Source: CAD feature listing. Evaluate the final solid. Frame: model axes, mm. Face numbers are marked on the shaded views. A direction names the side the tool comes from. Give positions to 0.01 mm unless a question says otherwise; leave off trailing zeros. Loops run counter-clockwise (first coordinate to the right, second up) from the corner with the lowest first, then second, coordinate; pieces in that order, holes last. Notation, with made-up numbers: (-25.5, 73.25) -> (-10.5, 73.25) arc R24 cw to (-10.5, 90.25) -> close; hole circle Ø4 at (-19, 31). An arc over 180 degrees is marked (long way). Return JSON: item names as keys, results as strings. Group by question number.
(1) Cut plane A-A on z = 0. Return loops of the section in (x, y), then the cut area to 3 significant figures.
(2) Pin query (flat end, axial travel): pin 1 (3 mm diameter, centred on y = 0, z = 0, fed in from +X). Return the tip coordinate at first contact, or that it passes through.
(3) Cut plane C-C on y = 4.25. Return loops of the section in (x, z), then the cut area to 3 significant figures.
(4) Ray query, line 1 (Y direction, x = 2.4, z = 0); line 2 (Z direction, x = 0.9, y = 0); line 3 (Z direction, x = 2.8, y = -3.75). Return the intervals inside material, ascending. Write a range as from..to.
(5) Draft query along Y for the marked faces 6, 7 and 8. Return one class per face: released by +Y, released by -Y, zero draft, split by the parting line, or undercut.
(6) Cut plane B-B on y = 0. Return loops of the section in (x, z), then the cut area to 3 significant figures.
(7) Access query for the marked faces 1, 2, 3, 4 and 5. Directions: +Z, -Z, +X, -X, +Y, -Y. A direction counts if a zero-diameter tool reaches every point of the face in a straight line with its end or side. Return the directions, or none.
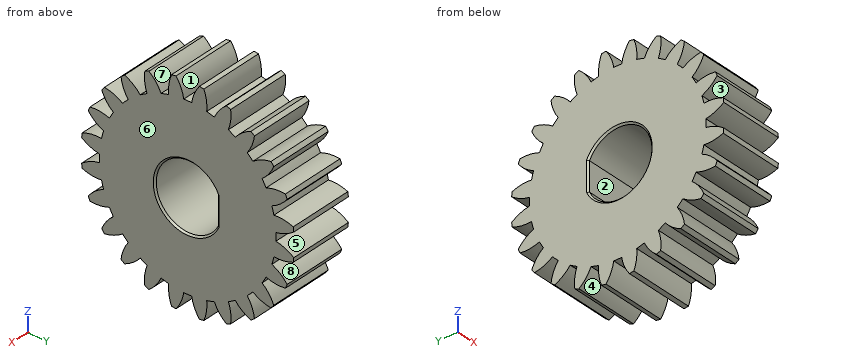
```python
from build123d import *

# Parameters (mm, degrees)
EXTRUDE_1_DEPTH = 4
CHAMFER_1_SIZE  = 0.1


with BuildPart() as part:
    # 草图1 → 凸台-拉伸1 (new body)
    with BuildSketch(Plane(origin=(0, 0, 0), x_dir=(0, -1, 0), z_dir=(-1, 0, 0))):
        with BuildLine():
            ThreePointArc((-0.711337602, 6.460959589), (-0.848420249, 6.444391599), (-0.98512003, 6.424915449))
            ThreePointArc((-0.98512003, 6.424915449), (-1.144628565, 5.84730165), (-1.156074481, 5.248177569))
            ThreePointArc((-1.156074481, 5.248177569), (-1.390893548, 5.19088539), (-1.622898915, 5.123092339))
            ThreePointArc((-1.622898915, 5.123092339), (-1.93237341, 5.636226055), (-2.359318752, 6.056700011))
            ThreePointArc((-2.359318752, 6.056700011), (-2.48744231, 6.005216961), (-2.614443361, 5.951023938))
            ThreePointArc((-2.614443361, 5.951023938), (-2.619019322, 5.351808006), (-2.475010506, 4.770136161))
            ThreePointArc((-2.475010506, 4.770136161), (-2.687, 4.65402052), (-2.893553842, 4.528490053))
            ThreePointArc((-2.893553842, 4.528490053), (-3.325292028, 4.944041268), (-3.846516229, 5.239686336))
            ThreePointArc((-3.846516229, 5.239686336), (-3.956949289, 5.156796712), (-4.065596697, 5.071579981))
            ThreePointArc((-4.065596697, 5.071579981), (-3.91492824, 4.49159749), (-3.625278654, 3.967017857))
            ThreePointArc((-3.625278654, 3.967017857), (-3.799991842, 3.799991842), (-3.967017857, 3.625278654))
            ThreePointArc((-3.967017857, 3.625278654), (-4.49159749, 3.91492824), (-5.071579981, 4.065596697))
            ThreePointArc((-5.071579981, 4.065596697), (-5.156796712, 3.956949289), (-5.239686336, 3.846516229))
            ThreePointArc((-5.239686336, 3.846516229), (-4.944041268, 3.325292028), (-4.528490053, 2.893553842))
            ThreePointArc((-4.528490053, 2.893553842), (-4.65402052, 2.687), (-4.770136161, 2.475010506))
            ThreePointArc((-4.770136161, 2.475010506), (-5.351808006, 2.619019322), (-5.951023938, 2.614443361))
            ThreePointArc((-5.951023938, 2.614443361), (-6.005216961, 2.48744231), (-6.056700011, 2.359318752))
            ThreePointArc((-6.056700011, 2.359318752), (-5.636226055, 1.93237341), (-5.123092339, 1.622898915))
            ThreePointArc((-5.123092339, 1.622898915), (-5.19088539, 1.390893548), (-5.248177569, 1.156074481))
            ThreePointArc((-5.248177569, 1.156074481), (-5.84730165, 1.144628565), (-6.424915449, 0.98512003))
            ThreePointArc((-6.424915449, 0.98512003), (-6.444391599, 0.848420249), (-6.460959589, 0.711337602))
            ThreePointArc((-6.460959589, 0.711337602), (-5.94431135, 0.407766737), (-5.368564348, 0.241646108))
            ThreePointArc((-5.368564348, 0.241646108), (-5.374, 0), (-5.368564348, -0.241646108))
            ThreePointArc((-5.368564348, -0.241646108), (-5.94431135, -0.407766737), (-6.460959589, -0.711337602))
            ThreePointArc((-6.460959589, -0.711337602), (-6.444391599, -0.848420249), (-6.424915449, -0.98512003))
            ThreePointArc((-6.424915449, -0.98512003), (-5.84730165, -1.144628565), (-5.248177569, -1.156074481))
            ThreePointArc((-5.248177569, -1.156074481), (-5.19088539, -1.390893548), (-5.123092339, -1.622898915))
            ThreePointArc((-5.123092339, -1.622898915), (-5.636226055, -1.93237341), (-6.056700011, -2.359318752))
            ThreePointArc((-6.056700011, -2.359318752), (-6.005216961, -2.48744231), (-5.951023938, -2.614443361))
            ThreePointArc((-5.951023938, -2.614443361), (-5.351808006, -2.619019322), (-4.770136161, -2.475010506))
            ThreePointArc((-4.770136161, -2.475010506), (-4.65402052, -2.687), (-4.528490053, -2.893553842))
            ThreePointArc((-4.528490053, -2.893553842), (-4.944041268, -3.325292028), (-5.239686336, -3.846516229))
            ThreePointArc((-5.239686336, -3.846516229), (-5.156796712, -3.956949289), (-5.071579981, -4.065596697))
            ThreePointArc((-5.071579981, -4.065596697), (-4.49159749, -3.91492824), (-3.967017857, -3.625278654))
            ThreePointArc((-3.967017857, -3.625278654), (-3.799991842, -3.799991842), (-3.625278654, -3.967017857))
            ThreePointArc((-3.625278654, -3.967017857), (-3.91492824, -4.49159749), (-4.065596697, -5.071579981))
            ThreePointArc((-4.065596697, -5.071579981), (-3.956949289, -5.156796712), (-3.846516229, -5.239686336))
            ThreePointArc((-3.846516229, -5.239686336), (-3.325292028, -4.944041268), (-2.893553842, -4.528490053))
            ThreePointArc((-2.893553842, -4.528490053), (-2.687, -4.65402052), (-2.475010506, -4.770136161))
            ThreePointArc((-2.475010506, -4.770136161), (-2.619019322, -5.351808006), (-2.614443361, -5.951023938))
            ThreePointArc((-2.614443361, -5.951023938), (-2.48744231, -6.005216961), (-2.359318752, -6.056700011))
            ThreePointArc((-2.359318752, -6.056700011), (-1.93237341, -5.636226055), (-1.622898915, -5.123092339))
            ThreePointArc((-1.622898915, -5.123092339), (-1.390893548, -5.19088539), (-1.156074481, -5.248177569))
            ThreePointArc((-1.156074481, -5.248177569), (-1.144628565, -5.84730165), (-0.98512003, -6.424915449))
            ThreePointArc((-0.98512003, -6.424915449), (-0.848420249, -6.444391599), (-0.711337602, -6.460959589))
            ThreePointArc((-0.711337602, -6.460959589), (-0.407766737, -5.94431135), (-0.241646108, -5.368564348))
            ThreePointArc((-0.241646108, -5.368564348), (0, -5.374), (0.241646108, -5.368564348))
            ThreePointArc((0.241646108, -5.368564348), (0.407766737, -5.94431135), (0.711337602, -6.460959589))
            ThreePointArc((0.711337602, -6.460959589), (0.848420249, -6.444391599), (0.98512003, -6.424915449))
            ThreePointArc((0.98512003, -6.424915449), (1.144628565, -5.84730165), (1.156074481, -5.248177569))
            ThreePointArc((1.156074481, -5.248177569), (1.390893548, -5.19088539), (1.622898915, -5.123092339))
            ThreePointArc((1.622898915, -5.123092339), (1.93237341, -5.636226055), (2.359318752, -6.056700011))
            ThreePointArc((2.359318752, -6.056700011), (2.48744231, -6.005216961), (2.614443361, -5.951023938))
            ThreePointArc((2.614443361, -5.951023938), (2.619019322, -5.351808006), (2.475010506, -4.770136161))
            ThreePointArc((2.475010506, -4.770136161), (2.687, -4.65402052), (2.893553842, -4.528490053))
            ThreePointArc((2.893553842, -4.528490053), (3.325292028, -4.944041268), (3.846516229, -5.239686336))
            ThreePointArc((3.846516229, -5.239686336), (3.956949289, -5.156796712), (4.065596697, -5.071579981))
            ThreePointArc((4.065596697, -5.071579981), (3.91492824, -4.49159749), (3.625278654, -3.967017857))
            ThreePointArc((3.625278654, -3.967017857), (3.799991842, -3.799991842), (3.967017857, -3.625278654))
            ThreePointArc((3.967017857, -3.625278654), (4.49159749, -3.91492824), (5.071579981, -4.065596697))
            ThreePointArc((5.071579981, -4.065596697), (5.156796712, -3.956949289), (5.239686336, -3.846516229))
            ThreePointArc((5.239686336, -3.846516229), (4.944041268, -3.325292028), (4.528490053, -2.893553842))
            ThreePointArc((4.528490053, -2.893553842), (4.65402052, -2.687), (4.770136161, -2.475010506))
            ThreePointArc((4.770136161, -2.475010506), (5.351808006, -2.619019322), (5.951023938, -2.614443361))
            ThreePointArc((5.951023938, -2.614443361), (6.005216961, -2.48744231), (6.056700011, -2.359318752))
            ThreePointArc((6.056700011, -2.359318752), (5.636226055, -1.93237341), (5.123092339, -1.622898915))
            ThreePointArc((5.123092339, -1.622898915), (5.19088539, -1.390893548), (5.248177569, -1.156074481))
            ThreePointArc((5.248177569, -1.156074481), (5.84730165, -1.144628565), (6.424915449, -0.98512003))
            ThreePointArc((6.424915449, -0.98512003), (6.444391599, -0.848420249), (6.460959589, -0.711337602))
            ThreePointArc((6.460959589, -0.711337602), (5.94431135, -0.407766737), (5.368564348, -0.241646108))
            ThreePointArc((5.368564348, -0.241646108), (5.374, 0), (5.368564348, 0.241646108))
            ThreePointArc((5.368564348, 0.241646108), (5.94431135, 0.407766737), (6.460959589, 0.711337602))
            ThreePointArc((6.460959589, 0.711337602), (6.444391599, 0.848420249), (6.424915449, 0.98512003))
            ThreePointArc((6.424915449, 0.98512003), (5.84730165, 1.144628565), (5.248177569, 1.156074481))
            ThreePointArc((5.248177569, 1.156074481), (5.19088539, 1.390893548), (5.123092339, 1.622898915))
            ThreePointArc((5.123092339, 1.622898915), (5.636226055, 1.93237341), (6.056700011, 2.359318752))
            ThreePointArc((6.056700011, 2.359318752), (6.005216961, 2.48744231), (5.951023938, 2.614443361))
            ThreePointArc((5.951023938, 2.614443361), (5.351808006, 2.619019322), (4.770136161, 2.475010506))
            ThreePointArc((4.770136161, 2.475010506), (4.65402052, 2.687), (4.528490053, 2.893553842))
            ThreePointArc((4.528490053, 2.893553842), (4.944041268, 3.325292028), (5.239686336, 3.846516229))
            ThreePointArc((5.239686336, 3.846516229), (5.156796712, 3.956949289), (5.071579981, 4.065596697))
            ThreePointArc((5.071579981, 4.065596697), (4.49159749, 3.91492824), (3.967017857, 3.625278654))
            ThreePointArc((3.967017857, 3.625278654), (3.799991842, 3.799991842), (3.625278654, 3.967017857))
            ThreePointArc((3.625278654, 3.967017857), (3.91492824, 4.49159749), (4.065596697, 5.071579981))
            ThreePointArc((4.065596697, 5.071579981), (3.956949289, 5.156796712), (3.846516229, 5.239686336))
            ThreePointArc((3.846516229, 5.239686336), (3.325292028, 4.944041268), (2.893553842, 4.528490053))
            ThreePointArc((2.893553842, 4.528490053), (2.687, 4.65402052), (2.475010506, 4.770136161))
            ThreePointArc((2.475010506, 4.770136161), (2.619019322, 5.351808006), (2.614443361, 5.951023938))
            ThreePointArc((2.614443361, 5.951023938), (2.48744231, 6.005216961), (2.359318752, 6.056700011))
            ThreePointArc((2.359318752, 6.056700011), (1.93237341, 5.636226055), (1.622898915, 5.123092339))
            ThreePointArc((1.622898915, 5.123092339), (1.390893548, 5.19088539), (1.156074481, 5.248177569))
            ThreePointArc((1.156074481, 5.248177569), (1.144628565, 5.84730165), (0.98512003, 6.424915449))
            ThreePointArc((0.98512003, 6.424915449), (0.848420249, 6.444391599), (0.711337602, 6.460959589))
            ThreePointArc((0.711337602, 6.460959589), (0.407766737, 5.94431135), (0.241646108, 5.368564348))
            ThreePointArc((0.241646108, 5.368564348), (0, 5.374), (-0.241646108, 5.368564348))
            ThreePointArc((-0.241646108, 5.368564348), (-0.407766737, 5.94431135), (-0.711337602, 6.460959589))
        make_face()
        with BuildLine():
            Line((-1.8, -0.871779789), (-1.8, 0.871779789))
            ThreePointArc((-1.8, 0.871779789), (2, 0), (-1.8, -0.871779789))
        make_face(mode=Mode.SUBTRACT)
    extrude(amount=-EXTRUDE_1_DEPTH)

    # 倒角1
    chamfer_1_edges = [part.edges().sort_by_distance(p)[0] for p in [
        (4, -2, 0),
        (4, 1.8, 0),
        (0, -2, 0),
        (0, 1.8, 0),
    ]]
    chamfer(chamfer_1_edges, length=CHAMFER_1_SIZE)


solid = part.part
```
Answers:
{
 "1": {"outline": "(0, -5.37) -> (4, -5.37) -> (4, -2.1) -> (3.9, -2) -> (0.1, -2) -> (0, -2.1) -> close; (0, 1.9) -> (0.1, 1.8) -> (3.9, 1.8) -> (4, 1.9) -> (4, 5.37) -> (0, 5.37) -> close", "area": "27.8 mm²"},
 "2": {"pin 1": "through"},
 "3": {"outline": "(0, -3.8) -> (4, -3.8) -> (4, 3.8) -> (0, 3.8) -> close", "area": "30.4 mm²"},
 "4": {"line 1": "-5.37..-2, 1.8..5.37", "line 2": "-5.37..-2, 2..5.37", "line 3": "-5.2..-4.16, -3.85..3.85, 4.16..5.2"},
 "5": {"face 6": "zero draft", "face 7": "undercut", "face 8": "released by +Y"},
 "6": {"outline": "(0, -5.37) -> (4, -5.37) -> (4, -2.1) -> (3.9, -2) -> (0.1, -2) -> (0, -2.1) -> close; (0, 2.1) -> (0.1, 2) -> (3.9, 2) -> (4, 2.1) -> (4, 5.37) -> (0, 5.37) -> close", "area": "27.0 mm²"},
 "7": {"face 1": "+Z, +X, -X", "face 2": "+X, -X", "face 3": "+X, -X, -Y", "face 4": "-Z, +X, -X", "face 5": "+X, -X, +Y"}
}
